Check sheet for the modelled part. Datum: model origin and axes. Units: mm. Round coordinates to 2 decimals unless told otherwise and drop trailing zeros. Order: outer loops, then holes, each group sorted by start corner. A loop starts at its lowest first (then second) coordinate and runs counter-clockwise, first axis right, second up. Notation, with made-up numbers: (-2, -27) -> (26, -27) arc R22 cw to (26, -13) -> close; hole circle Ø10 at (58, 56.25). An arc over 180 degrees is marked (long way). Answer in a Markdown table with one row per item.
from build123d import *

# Parameters (mm, degrees)
BOSS_EXTRUDE1_DEPTH = 4
FILLET1_R           = 1


with BuildPart() as part:
    # Sketch2 → Boss-Extrude1 (new body)
    with BuildSketch(Plane(origin=(0, 0, 0), x_dir=(-1, 0, 0), z_dir=(0, 1, 0))):
        Polygon((-4.690238769, 155), (67.247234081, 320), (334.267832537, 360), (296.347290812, 316.561271604), (20, 0), (0, 0), (-74.690238769, 0), (-74.690238769, 155), align=None)
        with BuildLine():
            Line((-41.790238769, 147.9), (-41.790238769, 122.1))
            ThreePointArc((-41.790238769, 122.1), (-39.690238769, 120), (-37.590238769, 122.1))
            Line((-37.590238769, 122.1), (-37.590238769, 147.9))
            ThreePointArc((-37.590238769, 147.9), (-39.690238769, 150), (-41.790238769, 147.9))
        make_face(mode=Mode.SUBTRACT)
        with BuildLine():
            Line((36.947560473, 232.737466349), (60.597560473, 222.426428574))
            ThreePointArc((60.597560473, 222.426428574), (63.36183099, 223.512158057), (62.276101506, 226.276428574))
            Line((62.276101506, 226.276428574), (38.626101506, 236.587466349))
            ThreePointArc((38.626101506, 236.587466349), (35.86183099, 235.501736865), (36.947560473, 232.737466349))
        make_face(mode=Mode.SUBTRACT)
        with BuildLine():
            Line((48.209761231, 147.9), (48.209761231, 122.1))
            ThreePointArc((48.209761231, 122.1), (50.309761231, 120), (52.409761231, 122.1))
            Line((52.409761231, 122.1), (52.409761231, 147.9))
            ThreePointArc((52.409761231, 147.9), (50.309761231, 150), (48.209761231, 147.9))
        make_face(mode=Mode.SUBTRACT)
        with BuildLine():
            Line((145.339473414, 324.519087967), (149.161695636, 299.003786336))
            ThreePointArc((149.161695636, 299.003786336), (151.549633624, 297.23807057), (153.31534939, 299.626008558))
            Line((153.31534939, 299.626008558), (149.493127167, 325.141310189))
            ThreePointArc((149.493127167, 325.141310189), (147.105189179, 326.907025955), (145.339473414, 324.519087967))
        make_face(mode=Mode.SUBTRACT)
        with BuildLine():
            Line((166.710229804, 218.087105004), (186.146285223, 201.120085532))
            ThreePointArc((186.146285223, 201.120085532), (189.109326203, 201.321053574), (188.908358161, 204.284094554))
            Line((188.908358161, 204.284094554), (169.472302741, 221.251114025))
            ThreePointArc((169.472302741, 221.251114025), (166.509261762, 221.050145983), (166.710229804, 218.087105004))
        make_face(mode=Mode.SUBTRACT)
    extrude(amount=BOSS_EXTRUDE1_DEPTH)

    # Fillet1
    fillet1_edges = [part.edges().sort_by_distance(p)[0] for p in [
        (-20, 2, 0),
        (74.690238769, 2, 0),
        (74.690238769, 2, 155),
        (4.690238769, 2, 155),
        (-67.247234081, 2, 320),
        (-334.267832537, 2, 360),
    ]]
    fillet(fillet1_edges, radius=FILLET1_R)


solid = part.part
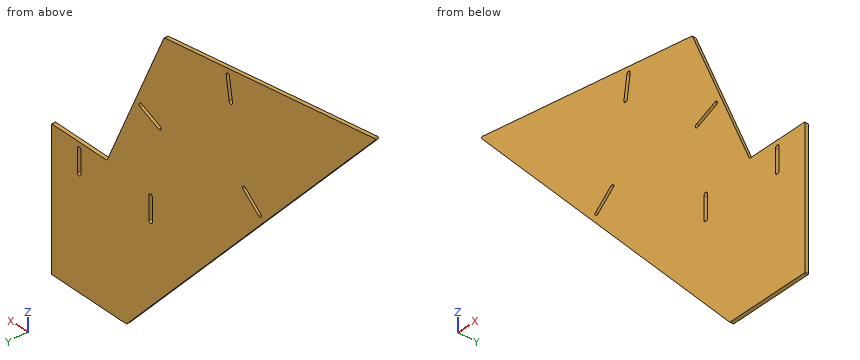
Item 1: Depth check by flat-ended pin: P1, Ø1.2, axis at y = 1, z = 132.5, coming from the -X side; P2, Ø1.5, axis at y = 2, z = 292, coming from the -X side; P3, Ø2, axis at y = 0.5, z = 125.5, coming from the -X side. Enter the tip coordinate at first touch or a pass-through.
Result sheet:
| item | result |
|---|---|
| P1 | stops at x = -136.19 |
| P2 | stops at x = -275.56 |
| P3 | stops at x = -130.43 |
Item 2: Cross-section at A-A (y = 0.95). State how many separate pieces and enclosed holes the cut face has, and give its area (3 significant figures).
Result sheet:
| item | result |
|---|---|
| separate pieces | 1 |
| enclosed holes | 5 |
| area | 61,500 mm^2 |
Item 3: Cross-section at C-C (x = -206). Record the boundary of the cut face in (y, z), and give its area (3 significant figures).
Result sheet:
| item | result |
|---|---|
| outline | (0, 213.07) -> (4, 213.07) -> (4, 340.79) -> (0, 340.79) -> close |
| area | 511 mm^2 |
Item 4: Cross-section at B-B (z = 29). Record the boundary of the cut face in (x, y), and give its area (3 significant figures).
Result sheet:
| item | result |
|---|---|
| outline | (-45.32, 0) -> (74.69, 0) -> (74.69, 4) -> (-45.32, 4) -> close |
| area | 480 mm^2 |
Item 5: Scan lines: line 1 (Z direction, x = -52, y = 1.65); line 2 (Z direction, x = -174, y = 3.8); line 3 (X direction, y = 0.45, z = 123). Record each from-to range of solid material in increasing order. Write a range as [from, to].
Result sheet:
| item | result |
|---|---|
| line 1 | z = [36.66, 120.85], [149.15, 226.17], [230.76, 285.03] |
| line 2 | z = [176.41, 211.72], [217.3, 335.99] |
| line 3 | x = [-127.37, -52.41], [-48.21, 37.59], [41.79, 74.69] |
